Build history of the part. All positions in model axes, mm. Give positions to 0.01 mm unless a question says otherwise; leave off trailing zeros. Loops run counter-clockwise (first coordinate to the right, second up) from the corner with the lowest first, then second, coordinate; pieces in that order, holes last. Notation, with made-up numbers: (-39.75, 68.25) -> (-2.75, 68.25) arc R25 cw to (-2.75, 94.25) -> close; hole circle Ø10 at (48.25, 78.5). An arc over 180 degrees is marked (long way). Answer as a JSON object with one key per item and string values. Group by question number.
Q1. Band-saw the part on A-A, the plane x = 7.5. Write the cut outline in (y, z).
Q2. Band-saw the part on B-B, the plane y = 0. Write the cut outline in (x, z).
Q3. Wall check: probe 1 along Y at (x, z) = (7.5, 2.5); probe 2 along X at (y, z) = (-1, 6.25); probe 3 along Z at (x, y) = (10.25, -15.5). Give the ranges that are in metal, low to high. Write a range as from..to.
Q4. Drop a flat-ended pin along its axis: pin 1 (3 mm diameter, centred on x = -1.99, z = 4.79, fed in from -Y). Give the stop position or say it passes through.
Q5. Band-saw the part on C-C, the plane x = -1.5. Write the cut outline in (y, z).
from build123d import *

# Parameters (mm, degrees)
SKETCH1_W          = 30
SKETCH1_H          = 46
EXTRUDE_3_8_DEPTH  = 9.63
SKETCH3_R          = 1.75
M4_DRILL_DEPTH     = 8
SKETCH5_R          = 2.25
CUT_EXTRUDE1_DEPTH = 10


with BuildPart() as part:
    # Sketch1 → 3/8 (new body)
    with BuildSketch(Plane.XY):
        Rectangle(SKETCH1_W, SKETCH1_H)
    extrude(amount=EXTRUDE_3_8_DEPTH)

    # Sketch3 → M4_DRILL (cut)
    with BuildSketch(Plane.XZ.offset(23)):
        with Locations(Location((-1.989909349, 4.787451112, 0), (0, 0, 270))):
            Circle(SKETCH3_R)
        with Locations(Location((10.005417301, 4.787451112, 0), (0, 0, 270))):
            Circle(SKETCH3_R)
    extrude(amount=-M4_DRILL_DEPTH, mode=Mode.SUBTRACT)

    # Sketch5 → Cut-Extrude1 (cut)
    with BuildSketch(Plane.XY.offset(9.63)):
        with Locations((7.5, 0)):
            Circle(SKETCH5_R)
    extrude(amount=-CUT_EXTRUDE1_DEPTH, mode=Mode.SUBTRACT)


solid = part.part
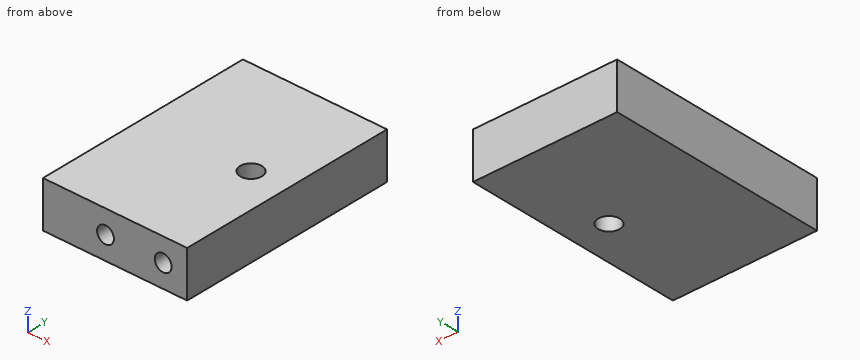
Worked answers:
{
 "1": {"outline": "(-23, 0) -> (-2.25, 0) -> (-2.25, 9.63) -> (-23, 9.63) -> close; (2.25, 0) -> (23, 0) -> (23, 9.63) -> (2.25, 9.63) -> close"},
 "2": {"outline": "(-15, 0) -> (5.25, 0) -> (5.25, 9.63) -> (-15, 9.63) -> close; (9.75, 0) -> (15, 0) -> (15, 9.63) -> (9.75, 9.63) -> close"},
 "3": {"probe 1": "-23..-2.25, 2.25..23", "probe 2": "-15..5.48, 9.52..15", "probe 3": "0..3.05, 6.52..9.63"},
 "4": {"pin 1": "y = -15"},
 "5": {"outline": "(-23, 0) -> (23, 0) -> (23, 9.63) -> (-23, 9.63) -> (-23, 6.47) -> (-15, 6.47) -> (-15, 3.11) -> (-23, 3.11) -> close"}
}
